from build123d import *

# Parameters (mm, degrees)
SKETCH1_W                      = 31.75
SKETCH1_H                      = 133.35
BOSS_EXTRUDE1_DEPTH            = 4.7625
M3X0_5_TAPPED_HOLE1_AT_2_COUNT = 2
M3X0_5_TAPPED_HOLE1_AT_2_PITCH = 19.05
F_12_0MM_DOWEL_HOLE1_D         = 12


with BuildPart() as part:
    # Sketch1 → Boss-Extrude1 (new, symmetric)
    with BuildSketch(Plane(origin=(0, 0, 0), x_dir=(0, 0, -1), z_dir=(1, 0, 0))):
        Rectangle(SKETCH1_W, SKETCH1_H)
    extrude(amount=BOSS_EXTRUDE1_DEPTH, both=True)

    # Sketch4 → M3x0.5 Tapped Hole1 (revolve, cut)
    with BuildSketch(Plane(origin=(0, 66.675, -9.525), x_dir=(0, 0, 1), z_dir=(1, 0, 0))):
        Polygon((0, 0), (0, 13.451075774), (1.25, 12.7), (1.25, 0), align=None)
    m3x0_5_tapped_hole1 = revolve(axis=Axis((0, 73.025, -9.525), (0, -1, 0)), mode=Mode.SUBTRACT)

    # M3x0.5 Tapped Hole1 at 2: M3x0.5 Tapped Hole1 ×2
    with Locations(*[(0, 0, i * M3X0_5_TAPPED_HOLE1_AT_2_PITCH) for i in range(1, M3X0_5_TAPPED_HOLE1_AT_2_COUNT)]):
        add(m3x0_5_tapped_hole1, mode=Mode.SUBTRACT)

    # Mirror1: M3x0.5 Tapped Hole1 across plane
    add(m3x0_5_tapped_hole1.mirror(Plane.ZX), mode=Mode.SUBTRACT)

    # Mirror1 copy 1 sketch → Mirror1 copy 1 (revolve, cut)
    with BuildSketch(Plane(origin=(0, -66.675, 9.525), x_dir=(0, 0, 1), z_dir=(1, 0, 0))):
        Polygon((0, 0), (0, -13.451075774), (1.25, -12.7), (1.25, 0), align=None)
    revolve(axis=Axis((0, -73.025, 9.525), (0, -1, 0)), mode=Mode.SUBTRACT)

    # Ø12.0mm Dowel Hole1 (through all)
    with Locations(Plane(origin=(4.7625, 0, 0), x_dir=(0, 0, -1), z_dir=(1, 0, 0))):
        with Locations((0, 0)):
            Hole(F_12_0MM_DOWEL_HOLE1_D / 2)


solid = part.part
The listing builds one solid part. Answer for the finished solid, in the listing's coordinates (mm). A direction names the side the tool comes from. Round coordinates to 2 decimals unless told otherwise and drop trailing zeros. Order: outer loops, then holes, each group sorted by start corner. A loop starts at its lowest first (then second) coordinate and runs counter-clockwise, first axis right, second up. Notation, with made-up numbers: (51.25, 16.25) -> (81.25, 16.25) arc R20 cw to (81.25, 55.25) -> close; hole circle Ø9 at (56, -11.75). An arc over 180 degrees is marked (long way). Write each question's results on one line, items separated by ' | '. Start each with the question number.
Q1. The mould has two halves that part along Z. Classify faces 1 (the flat face through (4.762, 1, -7)), 2 (the conical face through (0.083, 53.354, 9.726)), 3 (the flat face through (0, -1, 15.875)), 4 (the flat face through (0, -1, -15.875)): pulls with the +Z half, pulls with the -Z half, needs draft (parallel to the pull), parting line crosses it, or undercut.
Q2. Find section A-A (z = 0). Determine the outline of the cut face in (x, y) (1 decimal), then the cut area to 3 significant figures.
Q3. Which of the six approach directions +Z, -Z, +X, -X, +Y, -Y give full straight-line access (tool end or side, diameter ignored) to faces 5 (the cylindrical face through (1.22, 60.41, -9.8)), 6 (the cylindrical face through (1.22, -60.41, -9.8)), 7 (the flat face through (0, -66.675, 0))?
Q4. Straight lines are drawn through the part: probe 1 along Z at (x, y) = (0, 59.5) (3 decimals); probe 2 along Z at (x, y) = (-0.25, 4) (3 decimals); probe 3 along Y at (x, z) = (0.75, 1) (3 decimals). For each, find the intervals that lie inside material, in ascending order. Write a range as from..to.
Q5. Each of these flat-tipped pins is pushed along its axis until it touches: pin 1 (4 mm diameter, centred on x = 0, z = -9.525, fed in from +Y) (3 decimals); pin 2 (1.5 mm diameter, centred on x = 0, z = 9.525, fed in from +Y). Where does it stop, or does it pass through?
Q6. Find section C-C (x = 3.25). Determine the outline of the cut face in (y, z) (3 decimals).
Q7. Find section B-B (y = 0). Determine the outline of the cut face in (x, z) (1 decimal), then the cut area to 3 significant figures.
Worked answers:
1) face 1: needs draft | face 2: undercut | face 3: pulls with the +Z half | face 4: pulls with the -Z half
2) outline: (-4.8, -66.7) -> (4.8, -66.7) -> (4.8, -6) -> (-4.8, -6) -> close; (-4.8, 6) -> (4.8, 6) -> (4.8, 66.7) -> (-4.8, 66.7) -> close | area: 1,160 mm2
3) face 5: +Y | face 6: -Y | face 7: +Z, -Z, +X, -X, -Y
4) probe 1: z = -15.875..-10.775, -8.275..8.275, 10.775..15.875 | probe 2: z = -15.875..-4.472, 4.472..15.875 | probe 3: y = -66.675..-5.916, 5.916..66.675
5) pin 1: stops at y = 66.675 | pin 2: stops at y = 53.67
6) outline: (-66.675, -15.875) -> (66.675, -15.875) -> (66.675, 15.875) -> (-66.675, 15.875) -> close; hole circle Ø12 at (0, 0)
7) outline: (-4.8, -15.9) -> (4.8, -15.9) -> (4.8, -6) -> (-4.8, -6) -> close; (-4.8, 6) -> (4.8, 6) -> (4.8, 15.9) -> (-4.8, 15.9) -> close | area: 188 mm2
